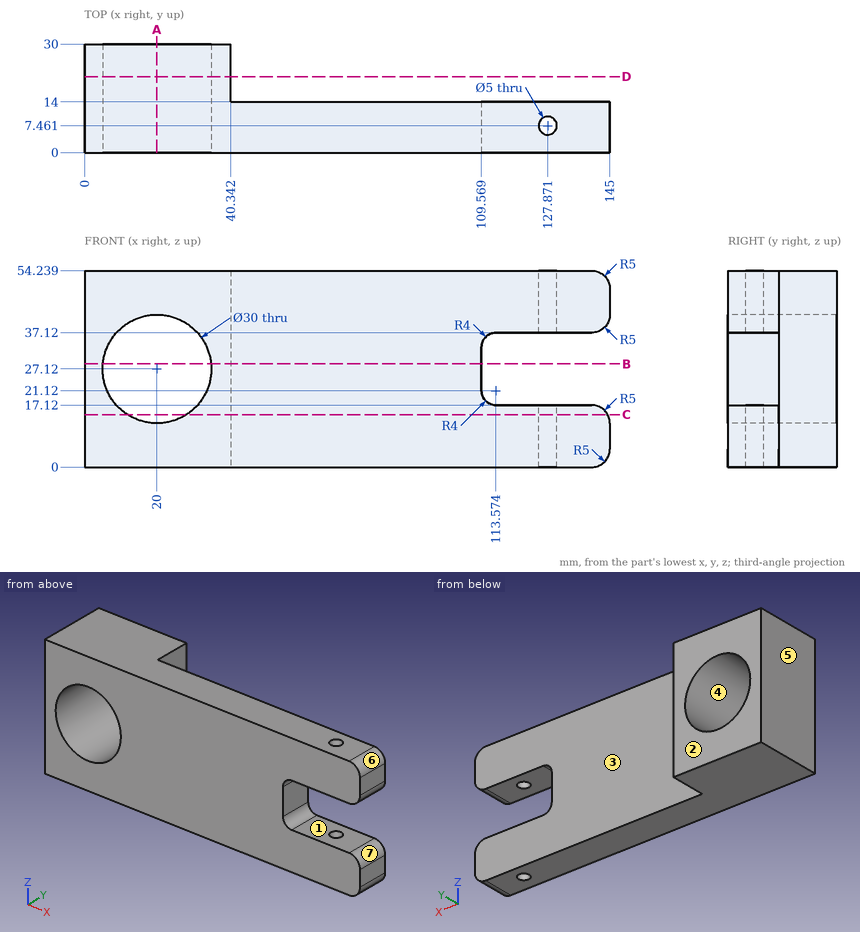
Part print with two shaded views. Sizes in mm from the minimum x, y, z corner. A direction names the side the tool comes from. Round coordinates to 2 decimals unless told otherwise and drop trailing zeros. Write each loop counter-clockwise with the first axis right and the second up, starting at its lowest first coordinate (ties: lowest second). Pieces come first, ordered by that corner, then holes. Notation, with made-up numbers: (12, 33) - (54, 33) arc R16 cw to (54, 53) - close; hole circle Ø10 at (74, -9.5). An arc over 180 degrees is marked (long way). Answer as CSV lines item,"result".
Q1. Cut at B-B (z = 28.5). Write the cut outline in (x, y).
Report:
outline,"(0, 0) - (5.06, 0) - (5.06, 30) - (0, 30) - close; (34.94, 0) - (109.57, 0) - (109.57, 14) - (40.34, 14) - (40.34, 30) - (34.94, 30) - close"
Q2. Drop flat-ended pins along their axis: pin 1 (13 mm diameter, centred on y = 24.5, z = 22.5, fed in from +X); pin 2 (5 mm diameter, centred on x = 122.5, z = 39, fed in from +Y); pin 3 (9.5 mm diameter, centred on y = 6, z = 26, fed in from +X). Give the stop position or say it passes through.
Report:
pin 1,"stops at x = 40.34"
pin 2,"stops at y = 14"
pin 3,"stops at x = 109.57"
Q3. Cut at C-C (z = 14.5). Write the cut outline in (x, y), and give its area (3 significant figures).
Report:
outline,"(0, 0) - (11.89, 0) - (11.89, 30) - (0, 30) - close; (28.11, 0) - (144.4, 0) - (144.4, 14) - (40.34, 14) - (40.34, 30) - (28.11, 30) - close; hole circle Ø5 at (127.87, 7.46)"
area,"2,160 mm^2"
Q4. Cut at D-D (y = 21). Write the cut outline in (x, z), and give its area (3 significant figures).
Report:
outline,"(0, 0) - (40.34, 0) - (40.34, 54.24) - (0, 54.24) - close; hole circle Ø30 at (20, 27.12)"
area,"1,480 mm^2"
Q5. Pull direction Z, two halves, no side cores. Call the marked faces 4, 5, 6 and 7: +Z half, -Z half, draft (parallel to the pull), parting line (faces both ways), or undercut.
Report:
face 4,"undercut"
face 5,"draft"
face 6,"+Z half"
face 7,"undercut"
Q6. Drill centre lines: probe 1 along Z at (x, y) = (123.5, 3.5); probe 2 along X at (y, z) = (28, 28) (1 decimal); probe 3 along X at (y, z) = (24, 3). Where is each one in solid material? Low to high. Write a range as [from, to].
Report:
probe 1,"z = [0, 17.12], [37.12, 54.24]"
probe 2,"x = [0, 5], [35, 40.3]"
probe 3,"x = [0, 40.34]"
Q7. Cut at A-A (x = 20). Write the cut outline in (y, z), and give its area (3 significant figures).
Report:
outline,"(0, 0) - (30, 0) - (30, 12.12) - (0, 12.12) - close; (0, 42.12) - (30, 42.12) - (30, 54.24) - (0, 54.24) - close"
area,"727 mm^2"
Q8. Tool access for the marked faces 1, 2 and 3: list every direction of +Z, -Z, +X, -X, +Y, -Y with a clear straight run to the whole face (end or side of a thin tool).
Report:
face 1,"+X, +Y, -Y"
face 2,"+Z, -Z, +X, -X, +Y"
face 3,"+Z, -Z, +X, +Y"
